Autodesk Inventor part; units mm, degrees
ref_plane "YZ Plane" through (0, 0, 0) normal (1, 0, 0) x (0, 1, 0)
ref_plane "XZ Plane" through (0, 0, 0) normal (0, 1, 0) x (-1, 0, 0)
ref_plane "XY Plane" through (0, 0, 0) normal (0, 0, 1) x (1, 0, 0)
sketch "Sketch2" plane through (0, 0, 0) normal (0, 1, 0) x (-1, 0, 0)
  line L0 (-89, 99) -> (89, 99)
  line L1 (89, 99) -> (89, -99)
  line L2 (89, -99) -> (-89, -99)
  line L3 (-89, -99) -> (-89, 99)
  line L4 (-89, 99) -> (89, -99) construction
  line L5 (89, 99) -> (-89, -99) construction
  line L6 (-89, 99) -> (89, 99)
  line L7 (89, 99) -> (89, -81)
  line L8 (89, -81) -> (-89, -81)
  line L9 (-89, -81) -> (-89, 99)
  line L10 (-4.5, 99) -> (-89, 99)
  line L11 (-89, 99) -> (-89, 46)
  line L12 (-89, 46) -> (-4.5, 46)
  line L13 (-4.5, 46) -> (-4.5, 99)
  line L14 (4.5, 99) -> (89, 99)
  line L15 (89, 99) -> (89, 46)
  line L16 (89, 46) -> (4.5, 46)
  line L17 (4.5, 46) -> (4.5, 99)
  line L18 (22.5, 77.5) -> (22.5, 66.5)
  line L19 (16.5, 66.5) -> (16.5, 77.5)
  line L20 (-22.5, 66.5) -> (-22.5, 77.5)
  line L21 (-16.5, 77.5) -> (-16.5, 66.5)
  line L22 (-22.5, 99) -> (-16.5, 99)
  line L23 (-16.5, 99) -> (-16.5, 46)
  line L24 (-16.5, 46) -> (-22.5, 46)
  line L25 (-22.5, 46) -> (-22.5, 99)
  line L26 (16.5, 99) -> (22.5, 99)
  line L27 (22.5, 99) -> (22.5, 46)
  line L28 (22.5, 46) -> (16.5, 46)
  line L29 (16.5, 46) -> (16.5, 99)
  line L30 (-89, 99) -> (89, 99)
  line L31 (89, 99) -> (89, 98)
  line L32 (89, 98) -> (-89, 98)
  line L33 (-89, 98) -> (-89, 99)
  line L34 (89, -81) -> (74, -81)
  line L35 (74, -81) -> (74, -65)
  line L36 (74, -65) -> (89, -65)
  line L37 (89, -65) -> (89, -81)
  line L38 (-89, -81) -> (-74, -81)
  line L39 (-74, -81) -> (-74, -65)
  line L40 (-74, -65) -> (-89, -65)
  line L41 (-89, -65) -> (-89, -81)
  point P0 (0, 0)
  point P1 (4.5, 99)
  point P2 (-4.5, 99)
  point P3 (-89, 46)
  point P4 (89, 46)
  point P5 (4.5, 98)
  point P6 (-4.5, 98)
  point P7 (-16.5, 98)
  point P8 (-22.5, 98)
  point P9 (22.5, 98)
  point P10 (16.5, 98)
  dimension "d8" = 178
  dimension "d9" = 198
  dimension "d10" = 18
  dimension "d11" = 84.5
  dimension "d12" = 53
  dimension "d13" = 84.5
  dimension "d14" = 53
  dimension "d17" = 9
  dimension "d18" = 1
  dimension "d19" = 15
  dimension "d20" = 16
  dimension "d21" = 15
  dimension "d22" = 16
extrude "Extrusion2" add sketch "Sketch2" along normal blind 3 contours L32 L23 L21 L12 L25 L20 | L12 L13 L32 L17 L16 L1 L36 L35 L8 L39 L40 L3 | L32 L27 L18 L16 L29 L19
equation "\"d11\" = d13"
properties part number "base" material "Aluminum 6061-AHC"
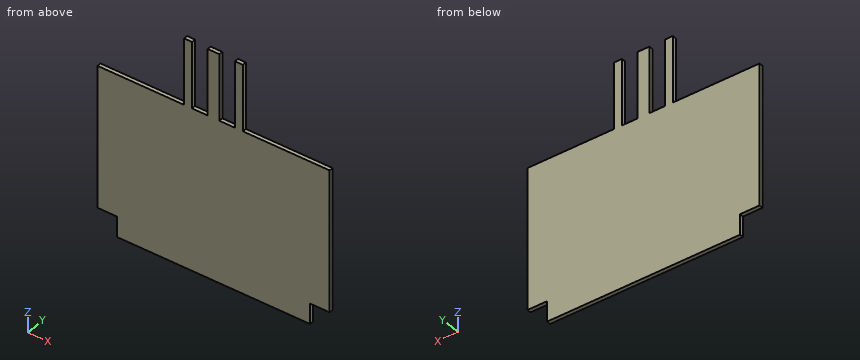
Can you work these out from the model? Positions are in its coordinate system, mm. Coordinates: 2 decimals unless noted, no trailing zeros. Loops run counter-clockwise (first coordinate to the right, second up) from the corner with the lowest first, then second, coordinate; pieces in that order, holes last. Notation, with made-up numbers: (65.25, -19.75) -> (119.25, -19.75) arc R23 cw to (119.25, 15.25) -> close; hole circle Ø5 at (-14, 43). An arc over 180 degrees is marked (long way). Put each result on its own line as item: value. Start each with the question number.
Q1. If I drill on line 1 (X direction, y = 1.75, z = 67); line 2 (Z direction, x = 77, y = 2.45); line 3 (X direction, y = 0.4, z = -71), over which ranges is the centre line in solid material (lowest first)? Write a range as [from, to].
Q2. I want a section at B-B (y = 2). Write out the boundary of the cut face in (x, z).
Q3. I'm going to push flat-ended pins straight in: P1, Ø1.5, axis at y = 2, z = 80, coming from the -X side; P2, Ø1.5, axis at x = -37.5, y = 1, coming from the +Z side; P3, Ø2, axis at x = 27.5, z = -10, coming from the -Y side; P4, Ø1.5, axis at y = 1, z = 79.5, coming from the +X side. Where does each tip first touch, or does it pass through?
Q4. I want a section at A-A (z = 65.5). Write out the boundary of the cut face in (x, y).
Q5. I want a section at C-C (x = -60.5). Write out the boundary of the cut face in (y, z), plus the area to 3 significant figures.
Taken from the geometry:
1. line 1: x = [-22.5, -16.5], [-4.5, 4.5], [16.5, 22.5]
1. line 2: z = [-65, 46]
1. line 3: x = [-74, 74]
2. outline: (-89, -65) -> (-74, -65) -> (-74, -81) -> (74, -81) -> (74, -65) -> (89, -65) -> (89, 46) -> (22.5, 46) -> (22.5, 98) -> (16.5, 98) -> (16.5, 46) -> (4.5, 46) -> (4.5, 98) -> (-4.5, 98) -> (-4.5, 46) -> (-16.5, 46) -> (-16.5, 98) -> (-22.5, 98) -> (-22.5, 46) -> (-89, 46) -> close
3. P1: stops at x = -22.5
3. P2: stops at z = 46
3. P3: stops at y = 0
3. P4: stops at x = 22.5
4. outline: (-22.5, 0) -> (-16.5, 0) -> (-16.5, 3) -> (-22.5, 3) -> close; (-4.5, 0) -> (4.5, 0) -> (4.5, 3) -> (-4.5, 3) -> close; (16.5, 0) -> (22.5, 0) -> (22.5, 3) -> (16.5, 3) -> close
5. outline: (0, -81) -> (3, -81) -> (3, 46) -> (0, 46) -> close
5. area: 381 mm2
